Part print with two shaded views. Sizes in mm from the minimum x, y, z corner. Coordinates: 2 decimals unless noted, no trailing zeros. Order: outer loops, then holes, each group sorted by start corner. A loop starts at its lowest first (then second) coordinate and runs counter-clockwise, first axis right, second up. Notation, with made-up numbers: (14, 4.25) - (34, 4.25) arc R16 cw to (34, 27.25) - close; hole circle Ø2 at (45.5, 5.5). An arc over 180 degrees is marked (long way). Return JSON: item names as keys, results as strings.
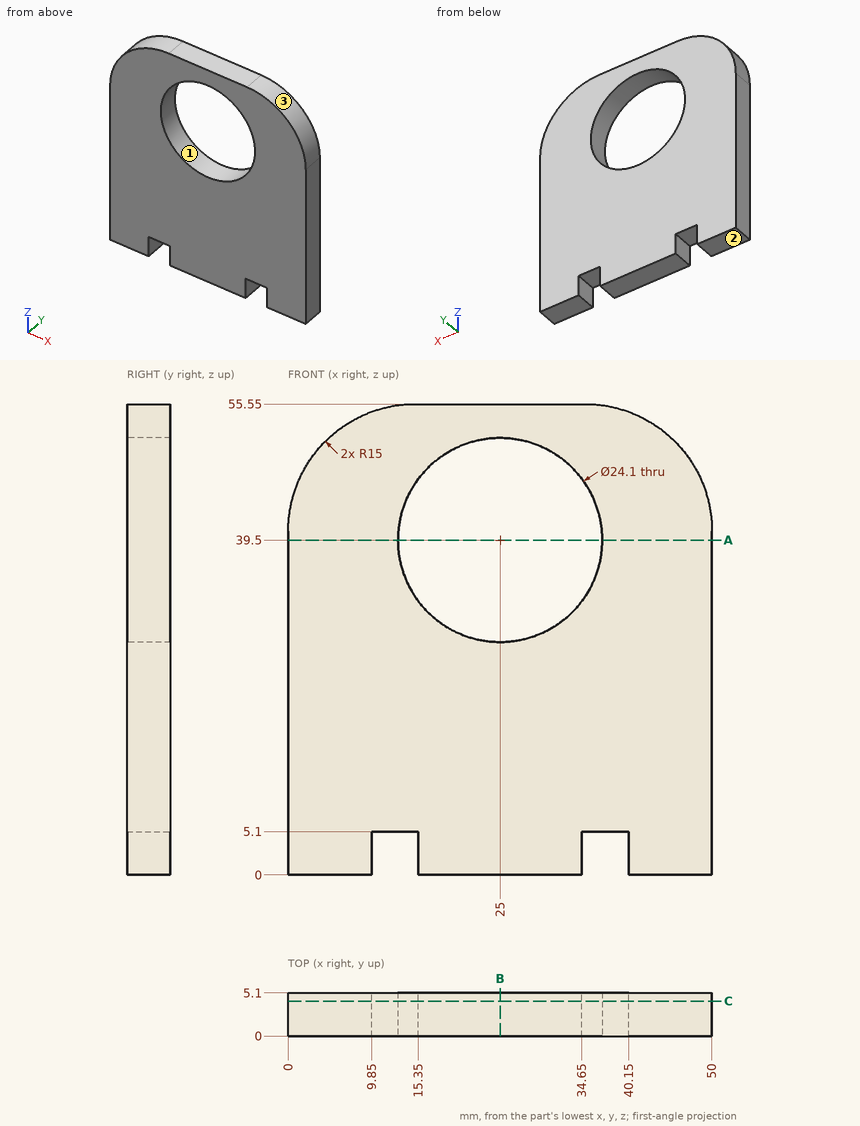
Item 1: Band-saw the part on A-A, the plane z = 39.5. List the corners of the cut face in (x, y).
Findings below:
{"outline": "(0, 0) - (12.95, 0) - (12.95, 5.1) - (0, 5.1) - close; (37.05, 0) - (50, 0) - (50, 5.1) - (37.05, 5.1) - close"}
Item 2: Band-saw the part on C-C, the plane y = 4.1. List the corners of the cut face in (x, z).
Findings below:
{"outline": "(0, 0) - (9.85, 0) - (9.85, 5.1) - (15.35, 5.1) - (15.35, 0) - (34.65, 0) - (34.65, 5.1) - (40.15, 5.1) - (40.15, 0) - (50, 0) - (50, 40.55) arc R15 ccw to (35, 55.55) - (15, 55.55) arc R15 ccw to (0, 40.55) - close; hole circle Ø24.1 at (25, 39.5)"}
Item 3: Wall check: L1, parallel to Z at x = 25, y = 2.45; L2, parallel to X at y = 2.1, z = 39.5; L3, parallel to X at y = 4.4, z = 34. Give the ranges that are in metal, low to high. Write a range as [from, to].
Findings below:
{"L1": "z = [0, 27.45], [51.55, 55.55]", "L2": "x = [0, 12.95], [37.05, 50]", "L3": "x = [0, 14.28], [35.72, 50]"}
Item 4: Drop a flat-ended pin along its axis: P1, Ø21.5, axis at x = 25, z = 39.5, coming from the -Y side. Give the stop position or say it passes through.
Findings below:
{"P1": "passes through"}
Item 5: Mould opens along X. For the marked faces 1, 2 and 3 say: released by +X, released by -X, zero draft, split by the parting line, or undercut.
Findings below:
{"face 1": "undercut", "face 2": "zero draft", "face 3": "released by +X"}
Item 6: Band-saw the part on B-B, the plane x = 25. List the corners of the cut face in (y, z).
Findings below:
{"outline": "(0, 0) - (5.1, 0) - (5.1, 27.45) - (0, 27.45) - close; (0, 51.55) - (5.1, 51.55) - (5.1, 55.55) - (0, 55.55) - close"}
